Design review of the part built by this model. Coordinates are the model's own, in mm. A direction names the side the tool comes from. Coordinates: 2 decimals unless noted, no trailing zeros. Loops run counter-clockwise (first coordinate to the right, second up) from the corner with the lowest first, then second, coordinate; pieces in that order, holes last. Notation, with made-up numbers: (3.5, 84.25) - (29.5, 84.25) arc R9 ccw to (29.5, 94.25) - close; hole circle Ø3 at (35.5, 4). An arc over 180 degrees is marked (long way). Return JSON: item names as keys, results as strings. Group by question number.
Autodesk Fusion 360 part; units mm, degrees
sketch "Skizze1" plane through (0, 0, 0) normal (0, 0, 1) x (1, 0, 0)
  line L0 (-75, 50) -> (-55, 50)
  line L1 (-55, 50) -> (-55, 35.3603)
  line L2 (-55, 35.3603) -> (-75, 35.3603)
  line L3 (-75, 35.3603) -> (-75, 50)
  line L4 (-69.4, 50) -> (-69.4, 35.3603)
  line L5 (-66.5, 50) -> (-66.5, 35.3603)
  dimension "d1" = 20
  dimension "d2" = 5.6
  dimension "d3" = 2.9
extrude "Extrusion1" add sketch "Skizze1" along normal blind 2.7 contours L0 L2 L3 L4 | L0 L1 L2 L5 makes body 1 at (-73.1333, 45.1201, 0) makes body 2 at (-62.6667, 45.1201, 0)
extrude "Extrusion2" add sketch "Skizze1" along normal blind 36.7 contours L0 L2 L4 L5 bodies 1 2
sketch "Skizze2" plane through (-69.4, 0, 0) normal (-1, 0, 0) x (0, -1, 0)
  line L0 (-50, 2.7) -> (-35.3603, 2.7)
  line L1 (-35.3603, 2.7) -> (-35.3603, 36.7)
  line L2 (-35.3603, 36.7) -> (-50, 36.7)
  line L3 (-50, 36.7) -> (-50, 2.7)
  line L4 (-42.6802, 2.7) -> (-42.6802, 36.7) construction
  line L5 (-50, 12.7) -> (-35.3603, 12.7) construction
  line L6 (-50, 2.7) -> (-35.3603, 2.7) construction
  circle A0 centre (-42.6802, 12.7) radius 3.15
  dimension "d8" = 10
  dimension "d9" = 6.3
extrude "Extrusion3" cut sketch "Skizze2" against normal blind 3 contours A0 bodies 1
fillet "Abrundung1" radius 5.5 2 edges at (-75, 50, 1.35) (-75, 35.3603, 1.35) on bodies 1
sketch "Skizze3" plane through (0, 0, 2.7) normal (0, 0, 1) x (-1, 0, 0)
  line L0 (55, -50) -> (66.5, -50)
  line L1 (66.5, -50) -> (66.5, -35.3603)
  line L2 (66.5, -35.3603) -> (55, -35.3603)
  line L3 (55, -35.3603) -> (55, -50)
  line L4 (66.5, -38.1003) -> (55, -38.1003)
  line L5 (55, -47.26) -> (66.5, -47.26)
  line L6 (57.5, -38.1003) -> (57.5, -35.3603)
  line L7 (57.5, -47.26) -> (57.5, -50)
  dimension "d14" = 2.74
  dimension "d15" = 2.74
  dimension "d16" = 9
  dimension "d17" = 9
extrude "Extrusion4" add sketch "Skizze3" along normal blind 9 contours L0 L1 L5 L7 | L1 L2 L4 L6 bodies 1
chamfer "Fase2" distance 9 angle 45 2 edges at (-57.5, 36.7303, 11.7) (-57.5, 48.63, 11.7) on bodies 1
fillet "Abrundung2" radius 1 2 edges at (-69.4, 50, 19.7) (-69.4, 35.3603, 19.7) on bodies 1
fillet "Abrundung3" radius 2 2 edges at (-55, 50, 1.35) (-55, 35.3603, 1.35) on bodies 1
equation "d6 = 34 mm + 2.7 mm"
equation "d18 = 15 mm - 2.7 mm - 3.3 mm"
Item 1: Add section B-B (x = -67.75). State the section outline as (y, z) points, then the cut area to 3 significant figures.
Item 2: Add section D-D (z = 31). State the section outline as (x, y) points, then the cut area to 3 significant figures.
Item 3: For faces 5 (the face through (-60, 43, 2.7)), 6 (the face through (-66, 35.36, 10)), 7 (the face through (-69.115, 35.661, 19.938)), 8 (the face through (-69.099, 49.715, 19.938)), list the 3-axis set-ups (+Z, -Z, +X, -X, +Y, -Y) from which the entire face can be reached by the end or side of a thin tool; tool diameter is ignored.
Item 4: Add section A-A (z = 12.7). State the section outline as (x, y) points.
Item 5: To check wall thickness, follow line 1 (Z direction, x = -69.5, y = 38); line 2 (X direction, y = 47.75, z = 34); line 3 (X direction, y = 49.25, z = 11.5). State the ranges of each line that lie inside material, in increasing order. Write a range as from..to.
Item 6: Draft analysis for pull direction Y (two halves, no side actions). For faces 1 (the face through (-55.57, 49.4, 1.37)), 2 (the face through (-66.5, 43, 23)), 3 (the face through (-61.9, 36.7, 7.1)), 4 (the face through (-63, 47.26, 6)), state which applies: pulls with the +Y half, pulls with the -Y half, needs draft (parallel to the pull), parting line crosses it, or undercut.
Item 7: Add section C-C (y = 40). State the section outline as (x, z) points (3 decimals).
Item 8: For P1, Ø4, axis at y = 39.5, z = 22, coming from the -X side; P2, Ø2, axis at x = -72.5, y = 46, coming from the +Z side; P3, Ø4, axis at y = 42.68, z = 12.7, coming from the +X side; P4, Ø8, axis at x = -58, y = 47.5, coming from the +Z side, all flat-tipped, find the tip position at first contact; note any pin that passes through.
Answers below:
{
 "1": {"outline": "(35.36, 0) - (50, 0) - (50, 36.7) - (35.36, 36.7) - close; hole circle Ø6.3 at (42.68, 12.7)", "area": "506 mm^2"},
 "2": {"outline": "(-69.4, 36.36) arc R1 ccw to (-68.4, 35.36) - (-66.5, 35.36) - (-66.5, 50) - (-68.4, 50) arc R1 ccw to (-69.4, 49) - close", "area": "42.0 mm^2"},
 "3": {"face 5": "+Z, +X", "face 6": "+Z, -Z, +X, -X, -Y", "face 7": "+Z, -X, -Y", "face 8": "+Z, -X, +Y"},
 "4": {"outline": "(-69.4, 36.36) arc R1 ccw to (-68.4, 35.36) - (-66.5, 35.36) - (-66.5, 39.53) - (-69.4, 39.53) - close; (-69.4, 45.83) - (-66.5, 45.83) - (-66.5, 50) - (-68.4, 50) arc R1 ccw to (-69.4, 49) - close"},
 "5": {"line 1": "z = 0..2.7", "line 2": "x = -69.4..-66.5", "line 3": "x = -69.37..-66.3"},
 "6": {"face 1": "pulls with the +Y half", "face 2": "undercut", "face 3": "needs draft", "face 4": "undercut"},
 "7": {"outline": "(-74.932, 0) - (-55, 0) - (-55, 2.7) - (-66.5, 2.7) - (-66.5, 11.045) - (-69.4, 11.045) - (-69.4, 2.7) - (-74.932, 2.7) - close; (-69.4, 14.355) - (-66.5, 14.355) - (-66.5, 36.7) - (-69.4, 36.7) - close"},
 "8": {"P1": "stops at x = -69.4", "P2": "stops at z = 2.7", "P3": "passes through", "P4": "stops at z = 7.2"}
}
